Here's the drawing with two shaded views (mm, measured from the low corner). I have some questions. A direction names the side the tool comes from. Round coordinates to 2 decimals unless told otherwise and drop trailing zeros. Loops run counter-clockwise (first coordinate to the right, second up) from the corner with the lowest first, then second, coordinate; pieces in that order, holes last.
(1) I want a section at C-C on y = 8. Write out the boundary of the cut face in (x, z), plus the area to 3 significant figures.
(2) I want a section at B-B on z = 31.5. Write out the boundary of the cut face in (x, y), plus the area to 3 significant figures.
(3) Which directions (+Z, -Z, +X, -X, +Y, -Y) give clear straight access to the entire face, cutting with the end or side of a thin tool? Please do the marked faces 4, 5, 6, 7 and 8.
(4) Thinking about a two-plate mould opening in X: for the marked faces 1, 2 and 3, which applies, released by +X, released by -X, zero draft, split by the parting line, or undercut?
(5) I want a section at A-A on y = 13. Write out the boundary of the cut face in (x, z).
(6) Will these pins go through, and if not, where does the flat tip stop? pin 1 Ø12 at (x, y) = (5.5, 19) entering from +Z; pin 2 Ø2.5 at (x, y) = (21, 2.5) entering from -Z (1 decimal); pin 3 Ø4 at (x, y) = (31, 4) entering from -Z.
(7) If I drill on line 1 along Z through (x, y) = (0.55, 18) (1 decimal); line 2 along X through (y, z) = (15.5, 31); line 3 along Y through (x, z) = (24.25, 31.35), over which ranges is the centre line in solid material (lowest first)?
(8) I want a section at D-D on x = 28.25. Write out the boundary of the cut face in (y, z).
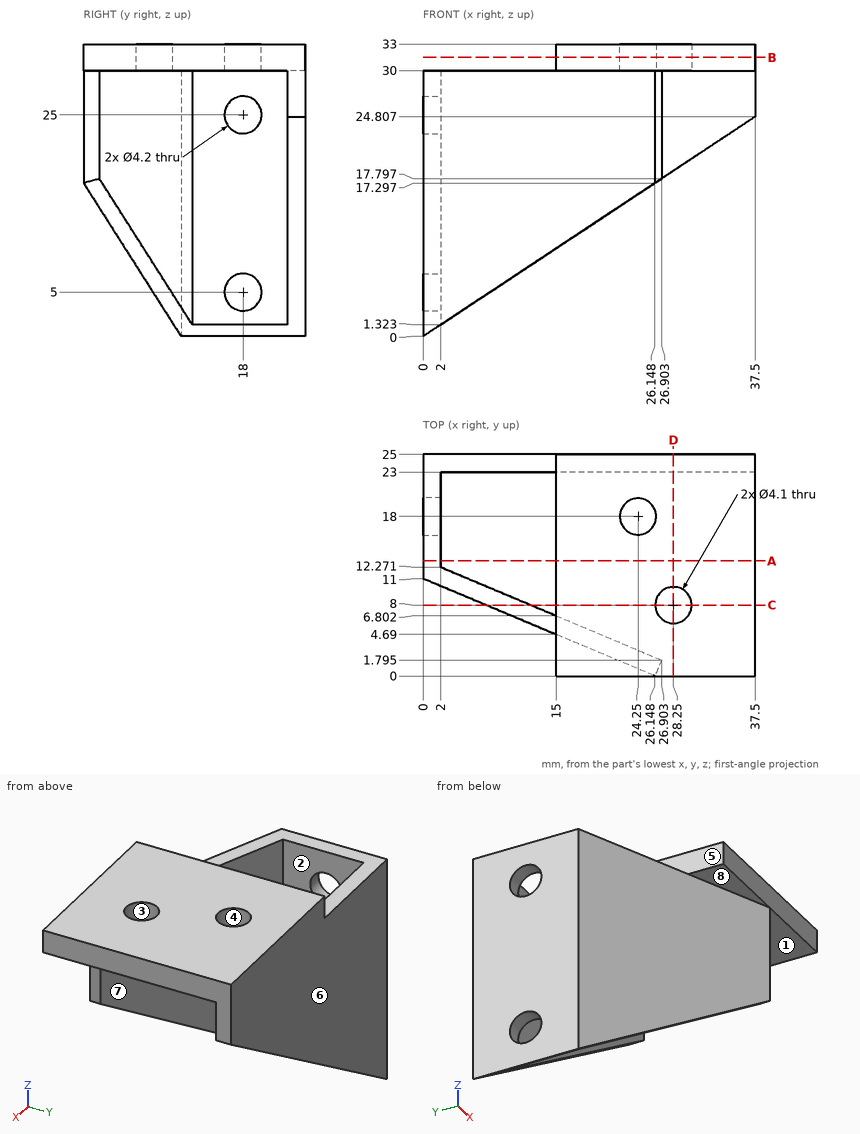
Filled sheet:
1. outline: (7.13, 4.72) - (12.15, 8.04) - (12.15, 30) - (7.13, 30) - close; (15, 30) - (26.2, 30) - (26.2, 33) - (15, 33) - close; (30.3, 30) - (37.5, 30) - (37.5, 33) - (30.3, 33) - close
1. area: 174 mm2
2. outline: (15, 0) - (37.5, 0) - (37.5, 25) - (15, 25) - close; hole circle Ø4.1 at (24.25, 18); hole circle Ø4.1 at (28.25, 8)
2. area: 536 mm2
3. face 4: +Z, -Z
3. face 5: +Z, -X, +Y, -Y
3. face 6: +Z, -Z, +X, -X, +Y
3. face 7: -Z, +X
3. face 8: -Z, -X, -Y
4. face 1: zero draft
4. face 2: released by +X
4. face 3: undercut
5. outline: (0, 0) - (2, 1.32) - (2, 30) - (0, 30) - close; (15, 30) - (37.5, 30) - (37.5, 33) - (15, 33) - close
6. pin 1: stops at z = 30
6. pin 2: stops at z = 13.1
6. pin 3: stops at z = 30
7. line 1: z = 0.4 to 2.9, 7.1 to 22.9, 27.1 to 30
7. line 2: x = 15 to 37.5
7. line 3: y = 0 to 15.95, 20.05 to 25
8. outline: (0, 30) - (5.95, 30) - (5.95, 33) - (0, 33) - close; (10.05, 30) - (23, 30) - (23, 18.69) - (25, 18.69) - (25, 33) - (10.05, 33) - close
